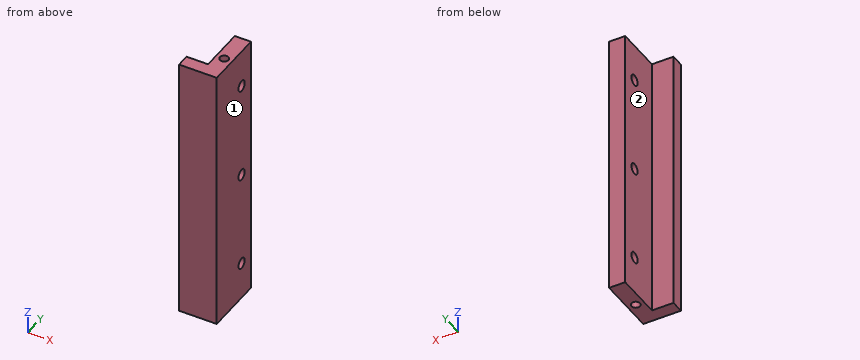
```python
from build123d import *

# Parameters (mm, degrees)
SKETCH_1_R                      = 4
EXTRUDE_1_DEPTH                 = 250
CUT_EXTRUDE_1_REACH             = 329.604
SKETCH_2_R                      = 5
CUT_EXTRUDE_1_DIRECTION_2_DEPTH = 328.604367435


with BuildPart() as part:
    # 草圖1 → 填料-伸長1 (new body)
    with BuildSketch(Plane.XY):
        Polygon((-5.019605957, 208.805223982), (-5.019605957, 165.805223982), (-25.019605957, 165.805223982), (-25.019605957, 153.805223982), (9.980394043, 153.805223982), (9.980394043, 208.805223982), align=None)
        with Locations((2.480394043, 178.805223982)):
            Circle(SKETCH_1_R, mode=Mode.SUBTRACT)
    extrude(amount=-EXTRUDE_1_DEPTH)

    # 草圖2 → 除料-伸長1 (cut, up to next)
    with BuildSketch(Plane(origin=(9.980394043, 0, 0), x_dir=(0, 0, -1), z_dir=(1, 0, 0)), mode=Mode.PRIVATE) as cut_extrude_1_sk1:
        with Locations(Location((35, 193.805223982, 0), (0, 0, 270))):
            Circle(SKETCH_2_R)
    cut_extrude_1_tool1 = extrude(cut_extrude_1_sk1.sketch, amount=-CUT_EXTRUDE_1_REACH, mode=Mode.PRIVATE) & part.part
    # 草圖2 → 除料-伸長1 (cut, up to next)
    with BuildSketch(Plane(origin=(9.980394043, 0, 0), x_dir=(0, 0, -1), z_dir=(1, 0, 0)), mode=Mode.PRIVATE) as cut_extrude_1_sk2:
        with Locations(Location((125, 193.805223982, 0), (0, 0, 270))):
            Circle(SKETCH_2_R)
    cut_extrude_1_tool2 = extrude(cut_extrude_1_sk2.sketch, amount=-CUT_EXTRUDE_1_REACH, mode=Mode.PRIVATE) & part.part
    # 草圖2 → 除料-伸長1 (cut, up to next)
    with BuildSketch(Plane(origin=(9.980394043, 0, 0), x_dir=(0, 0, -1), z_dir=(1, 0, 0)), mode=Mode.PRIVATE) as cut_extrude_1_sk3:
        with Locations(Location((215, 193.805223982, 0), (0, 0, 270))):
            Circle(SKETCH_2_R)
    cut_extrude_1_tool3 = extrude(cut_extrude_1_sk3.sketch, amount=-CUT_EXTRUDE_1_REACH, mode=Mode.PRIVATE) & part.part
    add(cut_extrude_1_tool1.solids().sort_by_distance((9.980394, 193.805224, -35))[0], mode=Mode.SUBTRACT)
    add(cut_extrude_1_tool2.solids().sort_by_distance((9.980394, 193.805224, -125))[0], mode=Mode.SUBTRACT)
    add(cut_extrude_1_tool3.solids().sort_by_distance((9.980394, 193.805224, -215))[0], mode=Mode.SUBTRACT)

    # 草圖2 → 除料-伸長1 direction 2 (cut)
    with BuildSketch(Plane(origin=(9.980394043, 0, 0), x_dir=(0, 0, -1), z_dir=(1, 0, 0))):
        with Locations(Location((35, 193.805223982, 0), (0, 0, 270))):
            Circle(SKETCH_2_R)
        with Locations(Location((125, 193.805223982, 0), (0, 0, 270))):
            Circle(SKETCH_2_R)
        with Locations(Location((215, 193.805223982, 0), (0, 0, 270))):
            Circle(SKETCH_2_R)
    extrude(amount=CUT_EXTRUDE_1_DIRECTION_2_DEPTH, mode=Mode.SUBTRACT)


solid = part.part
```
Check sheet for the modelled part. Datum: model origin and axes. Units: mm. Face numbers are marked on the shaded views. A direction names the side the tool comes from. Round coordinates to 2 decimals unless told otherwise and drop trailing zeros. Loops run counter-clockwise (first coordinate to the right, second up) from the corner with the lowest first, then second, coordinate; pieces in that order, holes last. Notation, with made-up numbers: (-6.5, 0.5) - (32.5, 0.5) arc R15 cw to (32.5, 28.5) - close; hole circle Ø11 at (-16, -15.5). An arc over 180 degrees is marked (long way). Answer as a JSON object with one key per item and string values. Group by question number.
Q1. Sectioned sample at C-C, the plane z = -193.5. Enter the section's corners in (x, y), plus the area to 3 significant figures.
Q2. Sectioned sample at A-A, the plane z = -35. Enter the section's corners in (x, y).
Q3. Sectioned sample at D-D, the plane y = 172. Enter the section's corners in (x, z).
Q4. Gauge pin test, flat ends, axial feed: P1, Ø8, axis at x = -12.5, z = -167.5, coming from the +Y side; P2, Ø2, axis at y = 171.5, z = -224.5, coming from the -X side. Record the tip position at first contact, or that the pin passes through.
Q5. Set-up check for the marked faces 1 and 2: record each of +Z, -Z, +X, -X, +Y, -Y from which the full face is reachable in a straight line by a thin tool's end or side.
Q6. Scan lines: line 1 along Y through (x, z) = (3, -125); line 2 along X through (y, z) = (178.5, -48); line 3 along Y through (x, z) = (0, -215). Record each from-to range of solid material in increasing order. Write a range as [from, to].
Q7. Sectioned sample at B-B, the plane y = 193.5. Enter the section's corners in (x, z).
Solution:
{
 "1": {"outline": "(-25.02, 153.81) - (9.98, 153.81) - (9.98, 208.81) - (-5.02, 208.81) - (-5.02, 165.81) - (-25.02, 165.81) - close; hole circle Ø8 at (2.48, 178.81)", "area": "1,010 mm²"},
 "2": {"outline": "(-25.02, 153.81) - (9.98, 153.81) - (9.98, 188.81) - (-5.02, 188.81) - (-5.02, 165.81) - (-25.02, 165.81) - close; (-5.02, 198.81) - (9.98, 198.81) - (9.98, 208.81) - (-5.02, 208.81) - close; hole circle Ø8 at (2.48, 178.81)"},
 "3": {"outline": "(-5.02, -250) - (9.98, -250) - (9.98, 0) - (-5.02, 0) - close"},
 "4": {"P1": "stops at y = 165.81", "P2": "stops at x = -5.02"},
 "5": {"face 1": "+Z, -Z, +X, +Y, -Y", "face 2": "+Z, -Z, -X, +Y"},
 "6": {"line 1": "y = [153.81, 174.84], [182.77, 188.81], [198.81, 208.81]", "line 2": "x = [-5.02, -1.51], [6.47, 9.98]", "line 3": "y = [153.81, 175.67], [181.94, 188.81], [198.81, 208.81]"},
 "7": {"outline": "(-5.02, -250) - (9.98, -250) - (9.98, -219.99) - (-5.02, -219.99) - close; (-5.02, -210.01) - (9.98, -210.01) - (9.98, -129.99) - (-5.02, -129.99) - close; (-5.02, -120.01) - (9.98, -120.01) - (9.98, -39.99) - (-5.02, -39.99) - close; (-5.02, -30.01) - (9.98, -30.01) - (9.98, 0) - (-5.02, 0) - close"}
}
